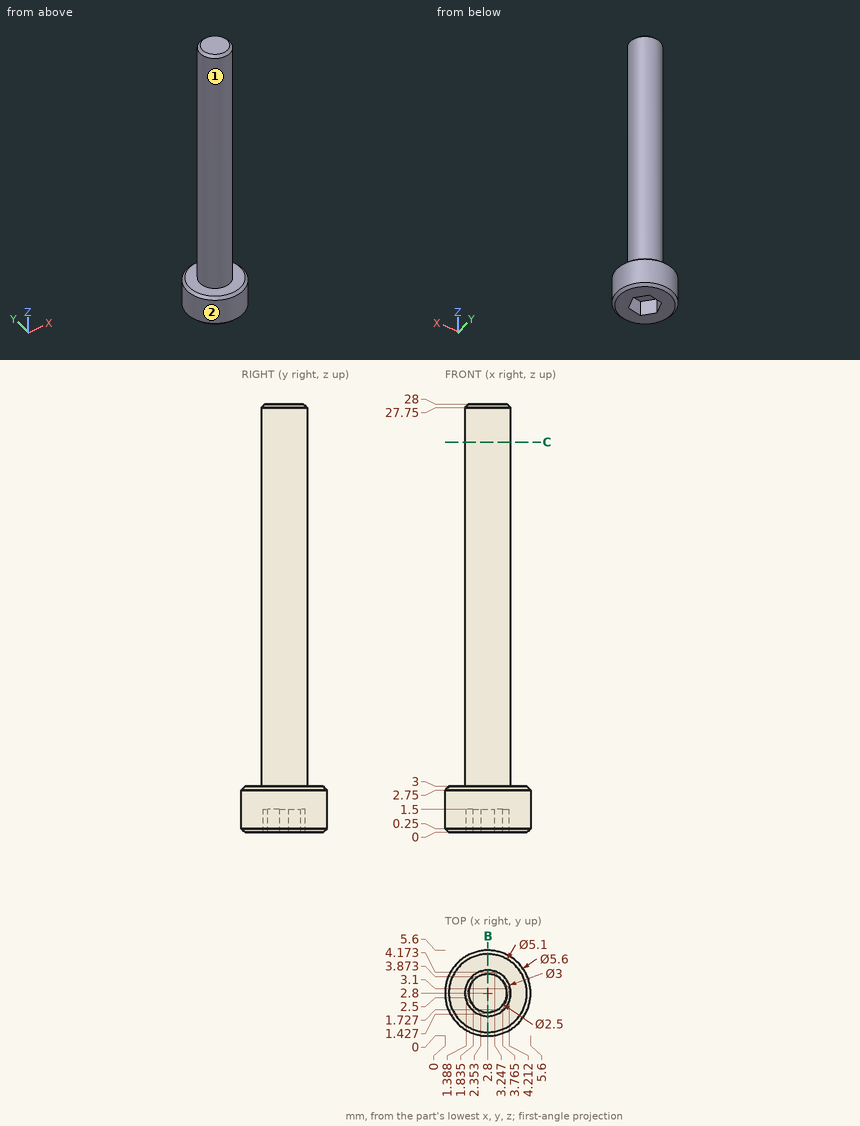
Geometry: see drawing. Coordinates: mm, zero at the bounding-box minimum. A direction names the side the tool comes from. Coordinates: 2 decimals unless noted, no trailing zeros. Write each loop counter-clockwise with the first axis right and the second up, starting at its lowest first coordinate (ties: lowest second). Pieces come first, ordered by that corner, then holes. Notation, with made-up numbers: (47, 86.5) - (55, 86.5) arc R17 ccw to (55, 115.5) - close; hole circle Ø6 at (47, 63). An arc over 180 degrees is marked (long way). Put each result on its own line as item: value. Start each with the question number.
1) Ray query, L1, parallel to Z at x = 1.2, y = 4.05; L2, parallel to Y at x = 2.75, z = 16. Return the intervals inside material, ascending.
2) Reachability of the marked faces 1 and 2 from +Z, -Z, +X, -X, +Y, -Y: full face, straight path, thin tool, end or side. Return the list, or none.
3) Cut plane C-C (z = 25.5). Return the cut outline in (x, y).
4) Cut plane B-B (x = 2.8). Return the cut outline in (y, z).
5) Contact query for flat-ended pins moving along their axis: pin 1 (3 mm diameter, centred on x = 4, z = 20.5, fed in from -Y); pin 2 (3 mm diameter, centred on x = 3, z = 20, fed in from +Y). Output: stop coordinate, or through.
Resolved:
1. L1: z = 0 to 3
1. L2: y = 1.3 to 4.3
2. face 1: +Z
2. face 2: +Z, -Z
3. outline: circle Ø3 at (2.8, 2.8)
4. outline: (0, 0.25) - (0.25, 0) - (1.52, 0) - (1.52, 1.5) - (4.08, 1.5) - (4.08, 0) - (5.35, 0) - (5.6, 0.25) - (5.6, 2.75) - (5.35, 3) - (4.3, 3) - (4.3, 27.75) - (4.05, 28) - (1.55, 28) - (1.3, 27.75) - (1.3, 3) - (0.25, 3) - (0, 2.75) - close
5. pin 1: stops at y = 1.3
5. pin 2: stops at y = 4.3
